Source: three-view drawing plus pictorial views. Frame: mm from the lowest corner of the part. A direction names the side the tool comes from. Round coordinates to 2 decimals unless told otherwise and drop trailing zeros. Write each loop counter-clockwise with the first axis right and the second up, starting at its lowest first coordinate (ties: lowest second). Pieces come first, ordered by that corner, then holes. Notation, with made-up numbers: (-7.75, 19) - (0.25, 19) arc R23 ccw to (0.25, 58) - close; hole circle Ø2 at (70, 9.5). An arc over 180 degrees is marked (long way). Write each question's results on one line, items separated by ' | '.
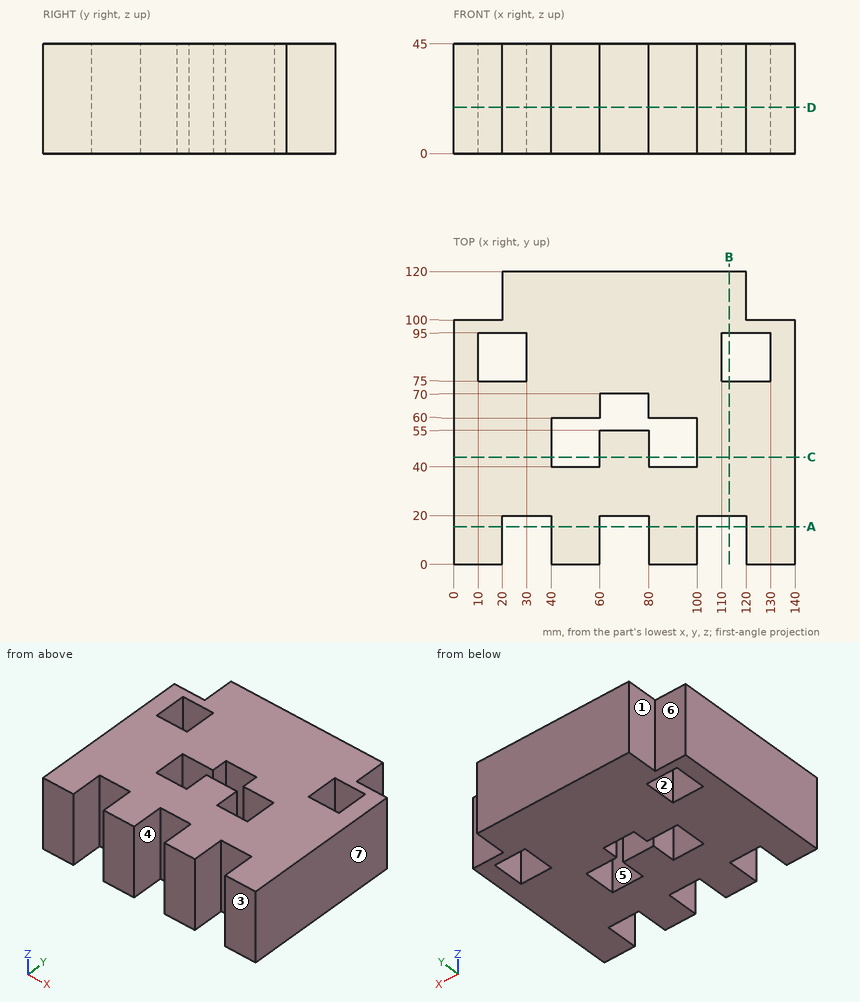
Q1. Ray query, line 1 along Y through (x, z) = (99, 29.5); line 2 along X through (y, z) = (83, 7); line 3 along X through (y, z) = (57, 25.5). Return the intervals inside material, ascending.
Answer block:
line 1: 0 to 40, 60 to 120 | line 2: 0 to 10, 30 to 110, 130 to 140 | line 3: 0 to 40, 100 to 140
Q2. Access query for the marked faces 1, 2, 3 and 4. Directions: +Z, -Z, +X, -X, +Y, -Y. A direction counts if a zero-diameter tool reaches every point of the face in a straight line with its end or side. Return the directions, or none.
Answer block:
face 1: +Z, -Z, -X, +Y | face 2: +Z, -Z | face 3: +Z, -Z, +X, -X, -Y | face 4: +Z, -Z, -Y
Q3. Pin query (flat end, axial travel): pin 1 (10 mm diameter, centred on x = 68.5, z = 32, fed in from -Y). Return the tip coordinate at first contact, or that it passes through.
Answer block:
pin 1: y = 20
Q4. Section query A-A, the plane y = 15.5. Return loops of the section in (x, z), plus the area to 3 significant figures.
Answer block:
outline: (0, 0) - (20, 0) - (20, 45) - (0, 45) - close; (40, 0) - (60, 0) - (60, 45) - (40, 45) - close; (80, 0) - (100, 0) - (100, 45) - (80, 45) - close; (120, 0) - (140, 0) - (140, 45) - (120, 45) - close | area: 3,600 mm2
Q5. Section query C-C, the plane y = 44. Return loops of the section in (x, z), plus the area to 3 significant figures.
Answer block:
outline: (0, 0) - (40, 0) - (40, 45) - (0, 45) - close; (60, 0) - (80, 0) - (80, 45) - (60, 45) - close; (100, 0) - (140, 0) - (140, 45) - (100, 45) - close | area: 4,500 mm2
Q6. Mould query, pull axis Y, two halves, no side actions, for the marked faces 5, 6 and 7. Classes: pulls with the +Y half, pulls with the -Y half, needs draft (parallel to the pull), parting line crosses it, or undercut.
Answer block:
face 5: undercut | face 6: pulls with the +Y half | face 7: needs draft
Q7. Section query B-B, the plane x = 113. Return loops of the section in (y, z), plus the area to 3 significant figures.
Answer block:
outline: (20, 0) - (75, 0) - (75, 45) - (20, 45) - close; (95, 0) - (120, 0) - (120, 45) - (95, 45) - close | area: 3,600 mm2
Q8. Section query D-D, the plane z = 19. Give the number of separate pieces and of enclosed holes in the cut face, plus the area to 3 significant figures.
Answer block:
separate pieces: 1 | enclosed holes: 3 | area: 12,900 mm2
